Work out the finished part from the listing and answer in its coordinate system (mm). Face numbers are marked on the shaded views. A direction names the side the tool comes from. Round coordinates to 2 decimals unless told otherwise and drop trailing zeros. Order: outer loops, then holes, each group sorted by start corner. A loop starts at its lowest first (then second) coordinate and runs counter-clockwise, first axis right, second up. Notation, with made-up numbers: (-29, 25.5) -> (-24, 25.5) arc R18 cw to (-24, 34.5) -> close; hole circle Ø8 at (73, 9.25). An arc over 180 degrees is marked (long way). Use one line per item in the form item = value.
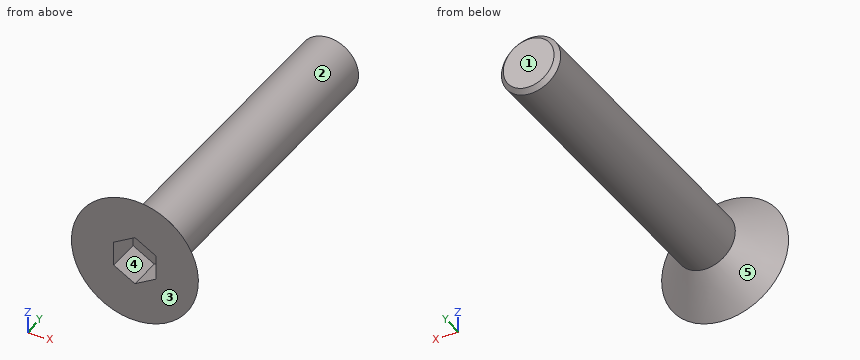
```python
from build123d import *

# Parameters (mm, degrees)
SKETCH_1_R      = 3
EXTRUDE_1_DEPTH = 1.6
CHAMFER_1_SIZE  = 1.6
SKETCH_2_R      = 1.4
EXTRUDE_2_DEPTH = 14.6
CHAMFER_2_SIZE  = 0.2


with BuildPart() as part:
    # 草图1 → 凸台-拉伸1 (new body)
    with BuildSketch(Plane(origin=(0, 0, 0), x_dir=(1, 0, 0), z_dir=(0, 1, 0))):
        with Locations(Location((0, 0, 0), (0, 0, 270))):
            Circle(SKETCH_1_R)
        Polygon((0, -1.154700538), (1, -0.577350269), (1, 0.577350269), (0, 1.154700538), (-1, 0.577350269), (-1, -0.577350269), align=None, mode=Mode.SUBTRACT)
    extrude(amount=EXTRUDE_1_DEPTH)

    # 倒角1
    # the kernel refuses this chamfer: 1.6 mm, written as the material it takes off along each edge
    with BuildSketch(Plane(origin=(0, 1.6, 0), x_dir=(0, 0, 1), z_dir=(-1, 0, 0))) as chamfer_1_piece_1:
        Polygon((3, -CHAMFER_1_SIZE), (3 - CHAMFER_1_SIZE, 0), (3, 0), align=None)
    revolve(axis=Axis((0, 1.6, 0), (0, 1, 0)), mode=Mode.SUBTRACT)

    # 草图2 → 凸台-拉伸2 (add)
    with BuildSketch(Plane(origin=(0, 1.6, 0), x_dir=(1, 0, 0), z_dir=(0, 1, 0))):
        with Locations(Location((0, 0, 0), (0, 0, 270))):
            Circle(SKETCH_2_R)
    extrude(amount=EXTRUDE_2_DEPTH)

    # 倒角2
    chamfer_2_edges = [part.edges().sort_by_distance(p)[0] for p in [
        (0, 16.2, -1.4),
    ]]
    chamfer(chamfer_2_edges, length=CHAMFER_2_SIZE)


solid = part.part
```
Item 1: Flat-ended cylindrical pins translate along their axes: P1, Ø1.3, axis at y = 0.5, z = -0.5, coming from the -X side; P2, Ø1.5, axis at y = 10, z = 0.5, coming from the -X side; P3, Ø2, axis at x = 1, y = 7, coming from the +Z side; P4, Ø1, axis at x = 2, y = 11.5, coming from the +Z side. Find the tip coordinate at first contact, or state that the pin passes through.
Findings:
P1 = -3
P2 = -1.4
P3 = 1.4
P4 = through
Item 2: Consider line 1 along X through (y, z) = (13.25, 0.1); line 2 along Y through (x, z) = (-0.7, -0.4); line 3 along Z through (x, y) = (-0.85, 13.75). Determine where each line is inside the solid, lowest interval first.
Findings:
line_1 = -1.4 to 1.4
line_2 = 1.6 to 16.2
line_3 = -1.11 to 1.11
Item 3: For the marked faces 1 and 2, determine the directions among +Z, -Z, +X, -X, +Y, -Y from which every point of the face is accessible in a straight line to the end or side of a thin tool.
Findings:
face_1 = +Z, -Z, +X, -X, +Y
face_2 = +Y
Item 4: The part is cut by section B-B, the plane y = 14.25. Give the vertices of the cut face in (x, z).
Findings:
outline = circle Ø2.8 at (0, 0)
Item 5: The part is cut by section A-A, the plane z = 0. Give the vertices of the cut face in (x, y), and give its area (3 significant figures).
Findings:
outline = (-3, 0) -> (-1, 0) -> (-1, 1.6) -> (1, 1.6) -> (1, 0) -> (3, 0) -> (1.4, 1.6) -> (1.4, 16) -> (1.2, 16.2) -> (-1.2, 16.2) -> (-1.4, 16) -> (-1.4, 1.6) -> close
area = 44.7 mm^2
Item 6: Determine the mould class of the marked faces 3, 4 and 5 for opening direction Z: released by +Z, released by -Z, zero draft, split by the parting line, or undercut.
Findings:
face_3 = zero draft
face_4 = undercut
face_5 = split by the parting line
